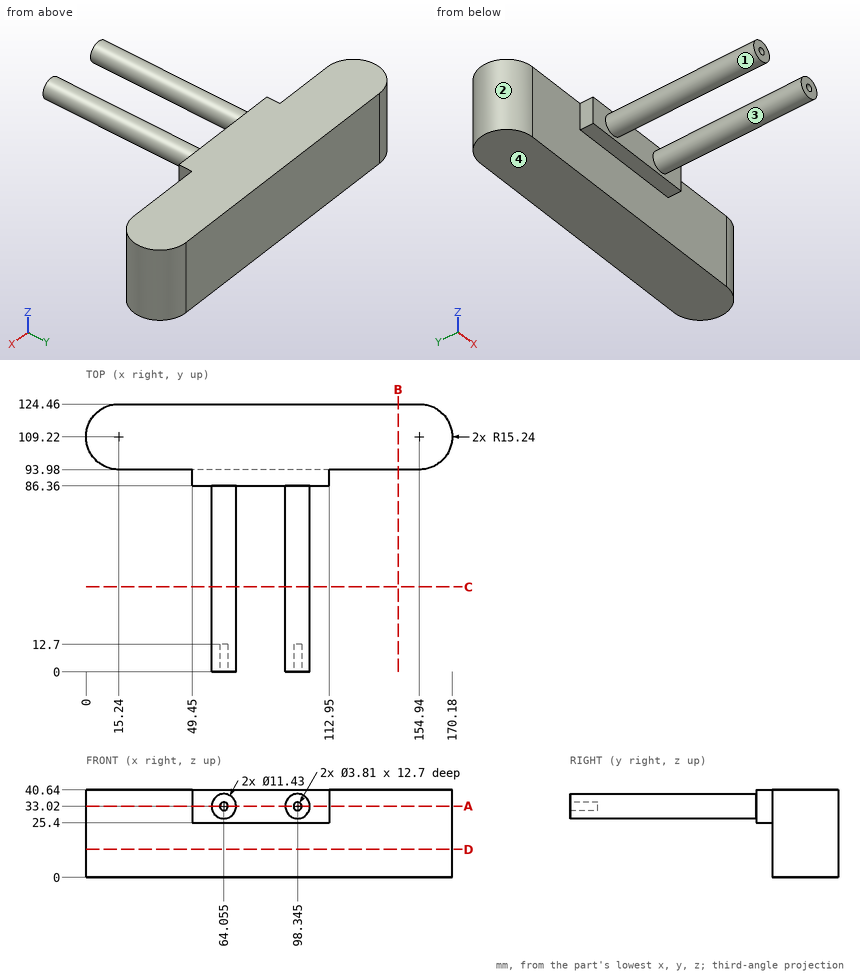
Geometry: see drawing. Coordinates: mm, zero at the bounding-box minimum. Give positions to 0.01 mm unless a question says otherwise; leave off trailing zeros. Write each loop counter-clockwise with the first axis right and the second up, starting at its lowest first coordinate (ties: lowest second). Pieces come first, ordered by that corner, then holes. Notation, with made-up numbers: M 5,-27.5 L 18,-27.5 A18 ccw 18,-16.5 Z; hole C -25.5,-38 d3. An arc over 180 degrees is marked long. Answer as a JSON object with one key per item and string values.
Q1. Contact query for flat-ended pins moving along their axis: P1, Ø4, axis at x = 87, y = 90, coming from the -Z side; P2, Ø2, axis at x = 21, z = 18, coming from the -Y side; P3, Ø8, axis at y = 79, z = 35.5, coming from the +X side. Output: stop coordinate, or through.
Geometry check:
{"P1": "stops at z = 25.4", "P2": "stops at y = 93.98", "P3": "stops at x = 104.06"}
Q2. Ray query, line 1 along X through (y, z) = (4, 33); line 2 along X through (y, z) = (67, 33); line 3 along Y through (x, z) = (148, 8). Return the intervals inside material, ascending.
Geometry check:
{"line 1": "x = 58.34 to 62.15, 65.96 to 69.77, 92.63 to 96.44, 100.25 to 104.06", "line 2": "x = 58.34 to 69.77, 92.63 to 104.06", "line 3": "y = 93.98 to 124.46"}
Q3. Cut plane D-D, the plane z = 13. Return the cut outline in (x, y).
Geometry check:
{"outline": "M 15.24,93.98 L 154.94,93.98 A15.24 ccw 154.94,124.46 L 15.24,124.46 A15.24 ccw Z"}
Q4. Cut plane B-B, the plane x = 145. Return the cut outline in (y, z), then the cut area to 3 significant figures.
Geometry check:
{"outline": "M 93.98,0 L 124.46,0 L 124.46,40.64 L 93.98,40.64 Z", "area": "1,240 mm^2"}
Q5. Cut plane C-C, the plane y = 39.5. Return the cut outline in (x, z) (3 decimals).
Geometry check:
{"outline": "C 64.055,33.02 d11.43; C 98.345,33.02 d11.43"}
Q6. Mould query, pull axis X, two halves, no side actions, for the marked faces 1, 2, 3 and 4. Classes: +X half, -X half, draft (parallel to the pull), parting line (faces both ways), or undercut.
Geometry check:
{"face 1": "undercut", "face 2": "-X half", "face 3": "undercut", "face 4": "draft"}
Q7. Cut plane A-A, the plane z = 33.02. Return the cut outline in (x, y), then the cut area to 3 significant figures.
Geometry check:
{"outline": "M 15.24,93.98 L 49.45,93.98 L 49.45,86.36 L 58.34,86.36 L 58.34,0 L 62.15,0 L 62.15,12.7 L 65.96,12.7 L 65.96,0 L 69.77,0 L 69.77,86.36 L 92.63,86.36 L 92.63,0 L 96.44,0 L 96.44,12.7 L 100.25,12.7 L 100.25,0 L 104.06,0 L 104.06,86.36 L 112.95,86.36 L 112.95,93.98 L 154.94,93.98 A15.24 ccw 154.94,124.46 L 15.24,124.46 A15.24 ccw Z", "area": "7,350 mm^2"}
